Could you check a few things on this model? Use its own coordinates, in mm. A direction names the side the tool comes from. Coordinates: 2 decimals unless noted, no trailing zeros. Loops run counter-clockwise (first coordinate to the right, second up) from the corner with the lowest first, then second, coordinate; pieces in that order, holes last. Notation, with made-up numbers: (20, 11) - (33, 11) arc R18 ccw to (33, 43) - close; hole circle Ø7 at (15, 37.25). An arc over 180 degrees is marked (long way). Put each result on its own line as item: value. Start each with the question number.
Autodesk Inventor part; units mm, degrees
ref_plane "YZ Plane" through (0, 0, 0) normal (1, 0, 0) x (0, 1, 0)
ref_plane "XZ Plane" through (0, 0, 0) normal (0, 1, 0) x (-1, 0, 0)
ref_plane "XY Plane" through (0, 0, 0) normal (0, 0, 1) x (1, 0, 0)
ref_plane "Work Plane1" through (47.167, -27.5147, -55.5227) normal (0, 1, 0) x (1, 0, 0)
sketch "Sketch1" plane through (47.167, -27.5147, -55.5227) normal (0, 1, 0) x (1, 0, 0)
  line L0 (-26, -54) -> (26, -54)
  line L1 (-26, 54) -> (-26, -54)
  line L2 (-26, -54) -> (26, -54)
  line L3 (26, -54) -> (26, 54)
  line L4 (26, 54) -> (-26, 54)
  line L5 (25.5, 53.5) -> (25.5, -53.5)
  line L6 (25.5, -53.5) -> (-25.5, -53.5)
  line L7 (-25.5, -53.5) -> (-25.5, 53.5)
  line L8 (-25.5, 53.5) -> (25.5, 53.5)
  line L9 (-24.5, -52.5) -> (24.5, -52.5)
  line L10 (24.5, -52.5) -> (24.5, 52.5)
  line L11 (24.5, 52.5) -> (-24.5, 52.5)
  line L12 (-24.5, 52.5) -> (-24.5, -52.5)
  line L13 (-24, -52) -> (-24, 52)
  line L14 (-24, 52) -> (24, 52)
  line L15 (24, 52) -> (24, -52)
  line L16 (24, -52) -> (-24, -52)
  point P0 (-47.167, -55.5227)
extrude "Extrusion1" add sketch "Sketch1" along normal blind 7.9375 contours L1 L4 L3 L0 | L5 L6 L7 L8 | L12 L11 L10 L9
sketch "Sketch2" plane through (47.167, -27.5147, -55.5227) normal (0, -1, 0) x (1, 0, 0)
  line L0 (-26, 54) -> (-26, -54)
  line L1 (-26, -54) -> (26, -54)
  line L2 (26, -54) -> (26, 54)
  line L3 (26, 54) -> (-26, 54)
  line L4 (-25, -53) -> (-25, 53) construction
  line L5 (-25, 53) -> (25, 53) construction
  line L6 (25, 53) -> (25, -53) construction
  line L7 (25, -53) -> (-25, -53) construction
  line L8 (-25.5, -53.5) -> (-25.5, 53.5)
  line L9 (-25.5, 53.5) -> (25.5, 53.5)
  line L10 (25.5, 53.5) -> (25.5, -53.5)
  line L11 (25.5, -53.5) -> (-25.5, -53.5)
  line L12 (-24.5, 52.5) -> (-24.5, -52.5)
  line L13 (-24.5, -52.5) -> (24.5, -52.5)
  line L14 (24.5, -52.5) -> (24.5, 52.5)
  line L15 (24.5, 52.5) -> (-24.5, 52.5)
  point P0 (-47.167, 55.5227)
  dimension "d2" = 1
  dimension "d3" = 1
extrude "Extrusion2" cut sketch "Sketch2" against normal blind 0.5 contours L8 L9 L10 L11
chamfer "Chamfer1" distance 0.25 angle 45 8 edges at (71.667, -27.0147, -55.5227) (47.167, -27.0147, -3.0227) (72.667, -27.0147, -55.5227) (47.167, -27.0147, -2.0227) (21.667, -27.0147, -55.5227) (22.667, -27.0147, -55.5227) (47.167, -27.0147, -108.0227) (47.167, -27.0147, -109.0227)
sketch "Sketch3" plane through (47.167, -19.5772, -55.5227) normal (0, 1, 0) x (1, 0, 0)
  line L0 (8, 26) -> (8, 24)
  line L1 (12, 24) -> (8, 24)
  line L2 (12, 48) -> (12, 24)
  line L3 (-12, 48) -> (12, 48)
  line L4 (-12, 24) -> (-12, 48)
  line L5 (-8, 24) -> (-12, 24)
  line L6 (-8, 24) -> (-8, 26)
  line L7 (-10, 26) -> (-8, 26)
  line L8 (-10, 46) -> (-10, 26)
  line L9 (10, 46) -> (-10, 46)
  line L10 (10, 26) -> (10, 46)
  line L11 (8, 26) -> (10, 26)
  line L12 (24, 52) -> (24, -52)
  line L13 (-24, 52) -> (24, 52)
  line L14 (-24, -52) -> (-24, 52)
  line L15 (24, -52) -> (-24, -52)
  line L16 (-8, 24) -> (8, 24)
  line L17 (8, 24) -> (8, 26)
  line L18 (8, 26) -> (-8, 26)
  line L19 (-8, 26) -> (-8, 24)
  point P0 (-47.167, -55.5227)
extrude "Extrusion3" add sketch "Sketch3" against normal blind 2 contours L11 L10 L9 L8 L7 L6 L5 L4 L3 L2 L1 L0 | L0 L16 L6 L18 | L12 L15 L14 L13
sketch "Sketch4" plane through (47.167, -19.5772, -55.5227) normal (0, 1, 0) x (1, 0, 0)
  line L0 (10, 26) -> (-10, 26)
  line L1 (-10, 26) -> (-10, 46)
  line L2 (-10, 46) -> (10, 46)
  line L3 (10, 46) -> (10, 26)
  line L4 (-26, -54) -> (26, -54)
  line L5 (26, -54) -> (26, 54)
  line L6 (26, 54) -> (-26, 54)
  line L7 (-26, 54) -> (-26, -54)
  line L8 (-12, 48) -> (-12, 24)
  line L9 (-12, 24) -> (12, 24)
  line L10 (12, 24) -> (12, 48)
  line L11 (12, 48) -> (-12, 48)
  point P0 (-47.167, -55.5227)
  dimension "d11" = 2
extrude "Extrusion4" add sketch "Sketch4" along normal blind 5.175 contours L11 L10 L9 L8
fillet "Fillet1" radius 4 4 edges at (47.167, -19.5772, -79.5227) (59.167, -19.5772, -91.5227) (47.167, -19.5772, -103.5227) (35.167, -19.5772, -91.5227)
equation "\"d2\" = 0.5 * outerShellThickness"
equation "\"d3\" = 0.5 * outerShellThickness"
equation "\"d9\" = outerShellThickness"
equation "\"d11\" = outerShellThickness"
equation "\"outerShellThickness\" = 2"
properties part number "Mid"
(1) Which directions (+Z, -Z, +X, -X, +Y, -Y) give clear straight access to the entire face, cutting with the end or side of a thin tool? Please do faces 4 (the flat face through (58, -14.402, -92)), 5 (the flat face through (48, -25, -3.523)), 6 (the flat face through (37.167, -18, -91)).
(2) I want a section at D-D on y = -24.5. List the corners of the cut face in (x, z) for me.
(3) I want a section at C-C on x = 29. List the corners of the cut face in (y, z) for me.
(4) If we mould it in two halves opening along X, with no side actions, what happens to faces 1 (the flat face through (71.167, -25, -56)), 2 (the flat face through (47, -24, -1.523)), 3 (the flat face through (73.167, -24, -55))? For each: pulls with the +X half, pulls with the -X half, needs draft (parallel to the pull), parting line crosses it, or undercut.
(5) I need wall thicknesses on L1, parallel to X at y = -22.5, z = -75; L2, parallel to Z at x = 65, y = -22.75; L3, parallel to Z at x = 50.5, y = -15.25. Which ranges of each line are inside material? Lowest first, please. Write a range as [from, to].
(6) For pin 1 Ø12 at (x, z) = (62, -52) entering from -Y; pin 2 Ø1.3 at (y, z) = (-15, -87) entering from +X; pin 3 Ø6 at (x, z) = (26.5, -41.5) entering from +Y, each with a flat end and sliding along its axis, tell me the tip position at first contact or that it passes through.
Answer sheet:
1. face 4: +Z, -Z, +X, -X, +Y
1. face 5: -Y
1. face 6: +Y, -Y
2. outline: (21.17, -109.52) - (73.17, -109.52) - (73.17, -1.52) - (21.17, -1.52) - close; hole (23.17, -107.52) - (71.17, -107.52) - (71.17, -3.52) - (23.17, -3.52) - close
3. outline: (-27.51, -109.52) - (-19.58, -109.52) - (-19.58, -1.52) - (-27.51, -1.52) - (-27.51, -2.02) - (-27.26, -2.02) - (-27.01, -2.27) - (-27.01, -2.77) - (-27.26, -3.02) - (-27.51, -3.02) - (-27.51, -3.52) - (-21.58, -3.52) - (-21.58, -107.52) - (-27.51, -107.52) - (-27.51, -108.02) - (-27.26, -108.02) - (-27.01, -108.27) - (-27.01, -108.77) - (-27.26, -109.02) - (-27.51, -109.02) - close
4. face 1: undercut
4. face 2: needs draft
4. face 3: pulls with the +X half
5. L1: x = [21.17, 23.17], [71.17, 73.17]
5. L2: z = [-109.52, -107.52], [-3.52, -1.52]
5. L3: z = [-103.52, -101.52], [-81.52, -79.52]
6. pin 1: stops at y = -21.58
6. pin 2: stops at x = 59.17
6. pin 3: stops at y = -19.58
